```python
from build123d import *

# Parameters (mm, degrees)
BASE_FLANGE1_DEPTH = 69.85
EDGE_FLANGE1_DEPTH = 276.04689029
EDGE_FLANGE3_DEPTH = 276.04689029
CUT_EXTRUDE1_REACH = 441.211
SKETCH16_W         = 8.739840912
SKETCH16_H         = 76.2


# Sheet-metal steps are written as plain solids
with BuildPart() as part:
    # Sketch1 → Base-Flange1 (new body)
    with BuildSketch(Plane(origin=(0, 0, 0), x_dir=(0, 0, -1), z_dir=(1, 0, 0))):
        with BuildLine():
            Line((0, 0), (0, 276.04689029))
            ThreePointArc((0, 276.04689029), (-0.056070336, 276.328774906), (-0.215745145, 276.567745145))
            Line((-0.215745145, 276.567745145), (-134.703841816, 411.055841816))
            Line((-134.703841816, 411.055841816), (-134.129105424, 411.630578208))
            Line((-134.129105424, 411.630578208), (0.358991247, 277.142481537))
            ThreePointArc((0.358991247, 277.142481537), (0.694858948, 276.63982), (0.8128, 276.04689029))
            Line((0.8128, 276.04689029), (0.8128, 0))
            Line((0.8128, 0), (0, 0))
        make_face()
    extrude(amount=BASE_FLANGE1_DEPTH)

    # Edge-Flange1 section (across the edge) → Edge-Flange1 (add)
    with BuildSketch(Plane(origin=(70.5866, 276.04689029, -0.8128), x_dir=(-1, 0, 0), z_dir=(0, -1, 0))):
        with BuildLine():
            Line((-0.8128, 0.7366), (-0.8128, 24.5872))
            Line((-0.8128, 24.5872), (0, 24.5872))
            Line((0, 24.5872), (0, 0.7366))
            ThreePointArc((0, 0.7366), (0.215745145, 0.215745145), (0.7366, 0))
            Line((0.7366, 0), (0.7366, -0.8128))
            ThreePointArc((0.7366, -0.8128), (-0.358991247, -0.358991247), (-0.8128, 0.7366))
        make_face()
    extrude(amount=EDGE_FLANGE1_DEPTH)

    # Edge-Flange3 section (across the edge) → Edge-Flange3 (add)
    with BuildSketch(Plane(origin=(-0.7366, 0, -0.8128), x_dir=(1, 0, 0), z_dir=(0, 1, 0))):
        with BuildLine():
            Line((-0.8128, 0.7366), (-0.8128, 62.6872))
            Line((-0.8128, 62.6872), (0, 62.6872))
            Line((0, 62.6872), (0, 0.7366))
            ThreePointArc((0, 0.7366), (0.215745145, 0.215745145), (0.7366, 0))
            Line((0.7366, 0), (0.7366, -0.8128))
            ThreePointArc((0.7366, -0.8128), (-0.358991247, -0.358991247), (-0.8128, 0.7366))
        make_face()
    extrude(amount=EDGE_FLANGE3_DEPTH)

    # Sketch16 → Cut-Extrude1 (cut, up to next)
    with BuildSketch(Plane.ZY.offset(1.5494), mode=Mode.PRIVATE) as cut_extrude1_sk1:
        with Locations((-59.130079544, 92.075)):
            Rectangle(SKETCH16_W, SKETCH16_H)
    cut_extrude1_tool1 = extrude(cut_extrude1_sk1.sketch, amount=-CUT_EXTRUDE1_REACH, mode=Mode.PRIVATE) & part.part
    add(cut_extrude1_tool1.solids().sort_by_distance((-1.5494, 92.075, -59.13008))[0], mode=Mode.SUBTRACT)


solid = part.part
```
The listing builds one solid part. Answer for the finished solid, in the listing's coordinates (mm). A direction names the side the tool comes from. Round coordinates to 2 decimals unless told otherwise and drop trailing zeros. Write each loop counter-clockwise with the first axis right and the second up, starting at its lowest first coordinate (ties: lowest second). Pieces come first, ordered by that corner, then holes. Notation, with made-up numbers: (-6, 25.25) -> (22, 25.25) arc R22 ccw to (22, 47.25) -> close; hole circle Ø1 at (53.5, 57). An arc over 180 degrees is marked (long way). Use CSV: the item, a comma, the result in double quotes. Start each with the question number.
(1) Consider L1, parallel to X at y = 228, z = -5; L2, parallel to Z at x = 23.5, y = 123; L3, parallel to X at y = 193, z = -52. Determine where each line is inside the solid, lowest interval first. Write a range as from..to.
(2) Section D-D on y = 171.5 is taken. Give the vertices of the cut face in (x, z), then the cut area to 3 significant figures.
(3) Each of these flat-tipped pins is pushed along its axis until it touches: pin 1 (21 mm diameter, centred on x = 42, y = 161, fed in from -Z); pin 2 (0.9 mm diameter, centred on x = -1.5, y = 98, fed in from -Z); pin 3 (1.7 mm diameter, centred on x = 70.5, z = -13.5, fed in from +Y). Where does it stop, or does it pass through?
(4) The mould has two halves that part along X. Classify faces 4 (the face through (34, 140, -0.813)), 5 (the face through (34.44, 342.87, 66.52)), 6 (the face through (71.399, 140, -13)), 7 (the face through (-0.737, 136, -33)): released by +X, released by -X, zero draft, split by the parting line, or undercut.
(5) Which of the six approach directions +Z, -Z, +X, -X, +Y, -Y give full straight-line access (tool end or side, diameter ignored) to faces 1 (the face through (70.587, 140, -14)), 2 (the face through (34, 136, 0)), 3 (the face through (34.4, 345.3, 67.8))?
(6) Section C-C on z = -44.5 is taken. Give the vertices of the cut face in (x, y), then the cut area to 3 significant figures.
(7) Section B-B on y = 72.5 is taken. Give the vertices of the cut face in (x, z).
(8) Section A-A on x = 53 is taken. Give the vertices of the cut face in (y, z).
A:
1,L1,"x = -1.55..-0.74, 70.59..71.4"
1,L2,"z = -0.81..0"
1,L3,"x = -1.55..-0.74"
2,outline,"(-1.55, -63.5) -> (-0.74, -63.5) -> (-0.74, -1.55) arc R0.74 cw to (0, -0.81) -> (69.85, -0.81) arc R0.74 cw to (70.59, -1.55) -> (70.59, -25.4) -> (71.4, -25.4) -> (71.4, -1.55) arc R1.55 ccw to (69.85, 0) -> (0, 0) arc R1.55 ccw to (-1.55, -1.55) -> close"
2,area,"129 mm²"
3,pin 1,"stops at z = -0.81"
3,pin 2,"stops at z = -54.76"
3,pin 3,"stops at y = 276.05"
4,face 4,"undercut"
4,face 5,"zero draft"
4,face 6,"released by +X"
4,face 7,"undercut"
5,face 1,"-Z, +Y, -Y"
5,face 2,"+Z, +X, -X, -Y"
5,face 3,"-Z, +X, -X, +Y"
6,outline,"(-1.55, 0) -> (-0.74, 0) -> (-0.74, 276.05) -> (-1.55, 276.05) -> close"
6,area,"224 mm²"
7,outline,"(-1.55, -54.76) -> (-0.74, -54.76) -> (-0.74, -1.55) arc R0.74 cw to (0, -0.81) -> (69.85, -0.81) arc R0.74 cw to (70.59, -1.55) -> (70.59, -25.4) -> (71.4, -25.4) -> (71.4, -1.55) arc R1.55 ccw to (69.85, 0) -> (0, 0) arc R1.55 ccw to (-1.55, -1.55) -> close"
8,outline,"(0, -0.81) -> (276.05, -0.81) arc R1.55 ccw to (277.14, -0.36) -> (411.63, 134.13) -> (411.06, 134.7) -> (276.57, 0.22) arc R0.74 cw to (276.05, 0) -> (0, 0) -> close"
